Could you check a few things on this model? Use its own coordinates, in mm. A direction names the side the tool comes from. Coordinates: 2 decimals unless noted, no trailing zeros. Order: outer loops, then holes, each group sorted by start corner. A loop starts at its lowest first (then second) coordinate and runs counter-clockwise, first axis right, second up. Notation, with made-up numbers: (24.25, 10.5) - (69.25, 10.5) arc R10 ccw to (69.25, 24.5) - close; hole circle Ø8 at (71.25, 31.25). An arc over 180 degrees is marked (long way). Answer as CSV lines item,"result". Start each with the question number.
1. For pin 1 (1 mm diameter, centred on x = 9, z = 3.5, fed in from +Y); pin 2 (4.5 mm diameter, centred on x = 0, y = 28.71, fed in from +Z); pin 3 (1 mm diameter, centred on x = 6.5, z = 2, fed in from +Y), each with a flat end and sliding along its axis, tell me the tip position at first contact or that it passes through.
2. I want a section at B-B, the plane x = 6. List the corners of the cut face in (y, z) for me.
3. I want a section at D-D, the plane y = -9.5. List the corners of the cut face in (x, z) for me, and give its area (3 significant figures).
4. I need wall thicknesses on probe 1 along Y at (x, z) = (0, 2.5); probe 2 along Z at (x, y) = (-4.5, 14.5); probe 3 along X at (y, z) = (5, 3.75). Which ranges of each line are inside material? Lowest first, please.
5. For faces 1 (the face through (0, 0, -1.5)), 2 (the face through (5.116, -0.988, 2.588)), which set-ups out of +Z, -Z, +X, -X, +Y, -Y let a thin tool reach every point of the face, with its end or its side?
6. I want a section at A-A, the plane x = 0. List the corners of the cut face in (y, z) for me (3 decimals).
7. Thinking about a two-plate mould opening in Y: for faces 3 (the face through (13.4, 34.43, -0.76)), 4 (the face through (-6.4, 0.5, 0)), 5 (the face through (0.2, 2.8, 1.8)), which applies, released by +Y, released by -Y, zero draft, split by the parting line, or undercut?
from build123d import *

# Parameters (mm, degrees)
SKETCH1_W           = 28
SKETCH1_H           = 70
BOSS_EXTRUDE1_DEPTH = 1.5
SKETCH3_R           = 6.941493401
BOSS_EXTRUDE2_DEPTH = 5.25
SKETCH2_R           = 2
SKETCH2_R_2         = 0.925
CUT_EXTRUDE1_DEPTH  = 39.295724304
FILLET1_R           = 2


with BuildPart() as part:
    # Sketch1 → Boss-Extrude1 (new body)
    with BuildSketch(Plane.XY):
        Rectangle(SKETCH1_W, SKETCH1_H)
    extrude(amount=-BOSS_EXTRUDE1_DEPTH)

    # Sketch3 → Boss-Extrude2 (add)
    with BuildSketch(Plane.XY):
        with Locations(Location((0, 3.703561495, 0), (0, 0, 180))):
            Circle(SKETCH3_R)
    extrude(amount=BOSS_EXTRUDE2_DEPTH)

    # Sketch2 → Cut-Extrude1 (cut, through all)
    with BuildSketch(Plane(origin=(0, 0, -1.5), x_dir=(-1, 0, 0), z_dir=(0, 0, -1))):
        with Locations((0.000493893, -21.295000553)):
            Circle(SKETCH2_R)
        with Locations((0.000493654, 28.705001831)):
            Circle(SKETCH2_R)
        with Locations((0, 3.703561495)):
            Circle(SKETCH2_R_2)
    extrude(amount=-CUT_EXTRUDE1_DEPTH, mode=Mode.SUBTRACT)

    # Fillet1
    fillet1_edges = [part.edges().sort_by_distance(p)[0] for p in [
        (14, 35, -0.75),
        (-14, 35, -0.75),
        (-14, -35, -0.75),
        (14, -35, -0.75),
    ]]
    fillet(fillet1_edges, radius=FILLET1_R)


solid = part.part
Solved:
1,pin 1,"passes through"
1,pin 2,"stops at z = 0"
1,pin 3,"stops at y = 7.19"
2,outline,"(-35, -1.5) - (35, -1.5) - (35, 0) - (7.19, 0) - (7.19, 5.25) - (0.21, 5.25) - (0.21, 0) - (-35, 0) - close"
3,outline,"(-14, -1.5) - (14, -1.5) - (14, 0) - (-14, 0) - close"
3,area,"42.0 mm2"
4,probe 1,"y = -3.24 to 2.78, 4.63 to 10.65"
4,probe 2,"z = -1.5 to 0"
4,probe 3,"x = -6.82 to 6.82"
5,face 1,"-Z, +X, -X, +Y, -Y"
5,face 2,"+Z"
6,outline,"(-35, -1.5) - (-23.295, -1.5) - (-23.295, 0) - (-35, 0) - close; (-19.295, -1.5) - (2.779, -1.5) - (2.779, 5.25) - (-3.238, 5.25) - (-3.238, 0) - (-19.295, 0) - close; (4.629, -1.5) - (26.705, -1.5) - (26.705, 0) - (10.645, 0) - (10.645, 5.25) - (4.629, 5.25) - close; (30.705, -1.5) - (35, -1.5) - (35, 0) - (30.705, 0) - close"
7,face 3,"released by +Y"
7,face 4,"zero draft"
7,face 5,"undercut"
